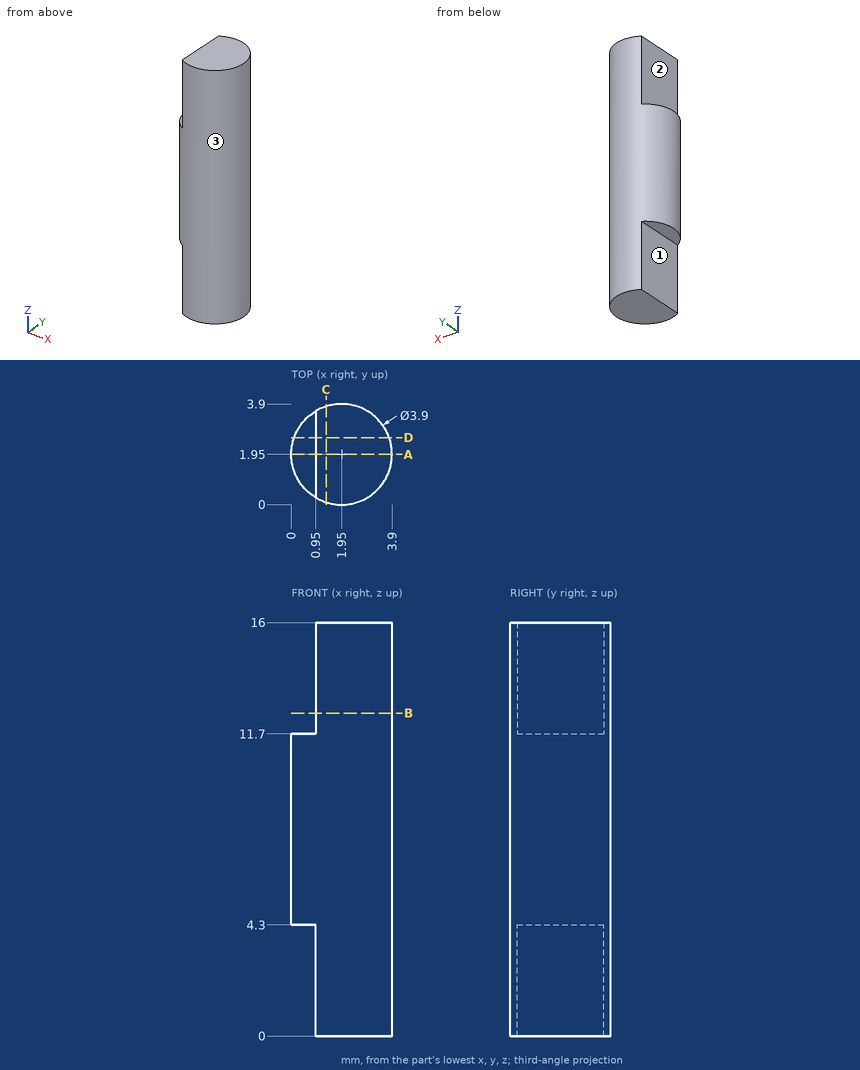
Source: three-view drawing plus pictorial views. Frame: mm from the lowest corner of the part. A direction names the side the tool comes from. Round coordinates to 2 decimals unless told otherwise and drop trailing zeros. Order: outer loops, then holes, each group sorted by start corner. A loop starts at its lowest first (then second) coordinate and runs counter-clockwise, first axis right, second up. Notation, with made-up numbers: (53, -22.75) -> (81, -22.75) arc R14 ccw to (81, -3.75) -> close; hole circle Ø3 at (18, -19.75). An arc over 180 degrees is marked (long way). Use one line per item in the form item = value. Start each with the question number.
1. Cut plane B-B (z = 12.5). Return the cut outline in (x, y), then the cut area to 3 significant figures.
2. Cut plane D-D (y = 2.6). Return the cut outline in (x, z).
3. Line query: probe 1 along X at (y, z) = (0.95, 2.25); probe 2 along Z at (x, y) = (0.7, 3.2); probe 3 along X at (y, z) = (2.2, 13.25). Output: solid intervals per line, ascending.
4. Cut plane A-A (y = 1.95). Return the cut outline in (x, z), then the cut area to 3 significant figures.
5. Pin query (flat end, axial travel): pin 1 Ø1 at (y, z) = (3.5, 7.5) entering from +X; pin 2 Ø1 at (y, z) = (1.5, 15) entering from -X; pin 3 Ø0.5 at (x, y) = (0.5, 2.5) entering from +Z. Return the tip coordinate at first contact, or that it passes through.
6. Cut plane C-C (x = 1.35). Return the cut outline in (y, z), then the cut area to 3 significant figures.
7. Reachability of the marked faces 1, 2 and 3 from +Z, -Z, +X, -X, +Y, -Y: full face, straight path, thin tool, end or side. Return the list, or none.
Solution:
q1.outline = (0.95, 0.28) arc R1.95 ccw (long way) to (0.95, 3.62) -> close
q1.area = 9.69 mm^2
q2.outline = (0.11, 4.3) -> (0.95, 4.3) -> (0.95, 0) -> (3.79, 0) -> (3.79, 16) -> (0.95, 16) -> (0.95, 11.7) -> (0.11, 11.7) -> close
q3.probe_1 = 0.95 to 3.62
q3.probe_2 = 4.3 to 11.7
q3.probe_3 = 0.95 to 3.88
q4.outline = (0, 4.3) -> (0.95, 4.3) -> (0.95, 0) -> (3.9, 0) -> (3.9, 16) -> (0.95, 16) -> (0.95, 11.7) -> (0, 11.7) -> close
q4.area = 54.2 mm^2
q5.pin_1 = 3.59
q5.pin_2 = 0.95
q5.pin_3 = 11.7
q6.outline = (0.09, 0) -> (3.81, 0) -> (3.81, 16) -> (0.09, 16) -> close
q6.area = 59.4 mm^2
q7.face_1 = -Z, -X, +Y, -Y
q7.face_2 = +Z, -X, +Y, -Y
q7.face_3 = +Z, -Z
